Design review of the part built by this model. Coordinates are the model's own, in mm. A direction names the side the tool comes from. Coordinates: 2 decimals unless noted, no trailing zeros. Loops run counter-clockwise (first coordinate to the right, second up) from the corner with the lowest first, then second, coordinate; pieces in that order, holes last. Notation, with made-up numbers: M 15.5,-4 L 29.5,-4 A28 ccw 29.5,19 Z; hole C 83.5,86.5 d6. An arc over 180 degrees is marked long. Put each result on its own line as item: value. Start each with the question number.
(1) Take a section at A-A, the plane x = 8. Give the boundary of the cut face in (y, z).
(2) Take a section at C-C, the plane y = 10. Count the separate pieces of the cut face and the enclosed holes in it, then the cut area to 3 significant figures.
(3) Take a section at B-B, the plane x = 18. Give the boundary of the cut face in (y, z), then the cut area to 3 significant figures.
(4) Clearance check with flat-ended pins moving along their axes: pin 1 (1.5 mm diameter, centred on y = 10, z = -42.5, fed in from +X); pin 2 (6.5 mm diameter, centred on x = 8, z = -25, fed in from -Y); pin 3 (9 mm diameter, centred on y = 14.5, z = -23, fed in from +X); pin 4 (1.5 mm diameter, centred on x = 23.5, y = 7.5, fed in from -Z). State where each tip first meets the part, or that it passes through.
(5) For faces 4 (the flat face through (16, 17, -25)), 5 (the flat face through (6, 12, -23)), 6 (the flat face through (20, 12, -25)), 7 (the cylindrical face through (56.88, 5.42, -12.58)), list the 3-axis set-ups (+Z, -Z, +X, -X, +Y, -Y) from which the entire face can be reached by the end or side of a thin tool; tool diameter is ignored.
(6) The part is to be moulded in two halves that separate along Z. For faces 1 (the flat face through (27, 0, -25)), 2 (the cylindrical face through (18, 18.4, -41.9)), 3 (the flat face through (11, 10, 0)), say which applies: +Z half, -Z half, draft (parallel to the pull), parting line (faces both ways), or undercut.
(7) For probe 1 along X at (y, z) = (13.7, -25); probe 2 along Z at (x, y) = (13.5, 3.75); probe 3 along Y at (x, z) = (15.5, -21.5), list the stretches that pass through material, from the lowest coordinate up. Write a range as [from, to].
```python
from build123d import *

# Parameters (mm, degrees)
EXTRUDE_1_DEPTH             = 20
SKETCH_2_R                  = 7
CUT_EXTRUDE_1_DEPTH         = 20
SKETCH_3_R                  = 13
CUT_EXTRUDE_2_DEPTH         = 87.740993769
SKETCH_4_R                  = 16
CUT_EXTRUDE_3_DEPTH         = 19
CUT_EXTRUDE_9_DEPTH         = 87.740993769
EXTRUDE_START               = -20
EXTRUDE_4_DEPTH             = 20
FILLET_2_R                  = 3
SKETCH_7_R                  = 20.5
CUT_EXTRUDE_10_DEPTH        = 9
SKETCH_8_W                  = 29.8
SKETCH_8_H                  = 4
CUT_EXTRUDE_11_DEPTH        = 20
CUT_EXTRUDE_12_DEPTH        = 10
HOLE_WIZARD_M41_D           = 4.3
HOLE_WIZARD_M41_DEPTH       = 8
HOLE_WIZARD_M41_CBORE_D     = 8
HOLE_WIZARD_M41_CBORE_DEPTH = 4.5
M4X0_71_D                   = 3.3
HOLE_WIZARD_M31_D           = 3.2


# Read off the part's stored shape, not the designer's step: Бобышка-Вытянуть4
with BuildPart() as part:
    # Эскиз1 → Бобышка-Вытянуть1 (new body)
    with BuildSketch(Plane(origin=(0, 0, 0), x_dir=(1, 0, 0), z_dir=(0, 1, 0))):
        with BuildLine():
            Line((0, 0), (0, 50))
            Line((0, 50), (20, 50))
            Line((20, 50), (47.60878471, 47.400960405))
            ThreePointArc((47.60878471, 47.400960405), (68, 25), (47.60878471, 2.599039595))
            Line((47.60878471, 2.599039595), (20, 0))
            Line((20, 0), (0, 0))
        make_face()
    extrude(amount=EXTRUDE_1_DEPTH)

    # Эскиз2 → Вырез-Вытянуть1 (cut)
    with BuildSketch(Plane.ZY):
        with Locations((-39.9, 10)):
            Circle(SKETCH_2_R)
        with Locations(Location((-10.1, 10, 0), (0, 0, 180))):
            Circle(SKETCH_2_R)
    extrude(amount=-CUT_EXTRUDE_1_DEPTH, mode=Mode.SUBTRACT)

    # Эскиз3 → Вырез-Вытянуть2 (cut, through all)
    with BuildSketch(Plane(origin=(0, 20, 0), x_dir=(1, 0, 0), z_dir=(0, 1, 0))):
        with Locations(Location((45.5, 25, 0), (0, 0, 270))):
            Circle(SKETCH_3_R)
    extrude(amount=-CUT_EXTRUDE_2_DEPTH, mode=Mode.SUBTRACT)

    # Эскиз4 → Вырез-Вытянуть3 (cut)
    with BuildSketch(Plane(origin=(0, 20, 0), x_dir=(1, 0, 0), z_dir=(0, 1, 0))):
        with Locations(Location((45.5, 25, 0), (0, 0, 270))):
            Circle(SKETCH_4_R)
    extrude(amount=-CUT_EXTRUDE_3_DEPTH, mode=Mode.SUBTRACT)

    # Эскиз5 → Вырез-Вытянуть9 (cut, through all)
    with BuildSketch(Plane(origin=(0, 20, 0), x_dir=(1, 0, 0), z_dir=(0, 1, 0))):
        with BuildLine():
            add(Edge.make_bspline(
                [(47.32108314, 47.428044097), (47.41641101, 47.41948544), (47.512308925, 47.410461109), (47.60878471, 47.400960405)],
                knots=[0.992066387, 0.992066387, 0.992066387, 0.992066387, 1, 1, 1, 1], degree=3))
            Line((47.32108314, 47.428044095), (47.60878471, 47.400960405))
        make_face()
        with BuildLine():
            Line((47.32108314, 47.428044097), (23, 49.717585585))
            add(Edge.make_bspline(
                [(23, 49.717585585), (32.393861284, 42.286998451), (35.400716473, 48.498269788), (47.32108314, 47.428044097)],
                knots=[0, 0, 0, 0, 0.992066387, 0.992066387, 0.992066387, 0.992066387], degree=3))
        make_face()
        with BuildLine():
            add(Edge.make_bspline(
                [(23, 0.282414415), (32.393861284, 7.713001549), (35.400716473, 1.501730212), (47.32108314, 2.571955903)],
                knots=[0, 0, 0, 0, 0.992066387, 0.992066387, 0.992066387, 0.992066387], degree=3))
            Line((23, 0.282414415), (47.32108314, 2.571955903))
        make_face()
        with BuildLine():
            Line((47.60878471, 2.599039595), (47.32108314, 2.571955905))
            add(Edge.make_bspline(
                [(47.32108314, 2.571955903), (47.41641101, 2.58051456), (47.512308925, 2.589538891), (47.60878471, 2.599039595)],
                knots=[0.992066387, 0.992066387, 0.992066387, 0.992066387, 1, 1, 1, 1], degree=3))
        make_face()
    extrude(amount=-CUT_EXTRUDE_9_DEPTH, mode=Mode.SUBTRACT)

    # Бобышка-Вытянуть4 outline → Бобышка-Вытянуть4 (add)
    with BuildSketch(Plane(origin=(0, 20, 0), x_dir=(1, 0, 0), z_dir=(0, 1, 0)).offset(EXTRUDE_START)):
        with BuildLine():
            add(Edge.make_bspline(
                [(22.6429674, 50), (22.761978267, 49.905861862), (22.880989133, 49.811723723), (23, 49.717585585)],
                knots=[-0.012568493, -0.012568493, -0.012568493, -0.012568493, 0, 0, 0, 0], degree=3))
            Line((22.6429674, 50), (20, 50))
            Line((20, 50), (23, 49.717585585))
        make_face()
        with BuildLine():
            Line((20, 0), (22.6479861, 0))
            add(Edge.make_bspline(
                [(22.6479861, 0), (22.766323231, 0.09625734), (22.883651508, 0.190382227), (23, 0.282414415)],
                knots=[-0.012287325, -0.012287325, -0.012287325, -0.012287325, 0, 0, 0, 0], degree=3))
            Line((23, 0.282414415), (20, 0))
        make_face()
    extrude(amount=EXTRUDE_4_DEPTH)

    # Скругление2
    fillet_2_edges = [part.edges().sort_by_distance(p)[0] for p in [
        (11.32399305, 0, 0),
        (11.32399305, 20, 0),
        (11.3214837, 0, -50),
        (11.3214837, 20, -50),
    ]]
    fillet(fillet_2_edges, radius=FILLET_2_R)

    # Эскиз7 → Вырез-Вытянуть10 (cut)
    with BuildSketch(Plane(origin=(0, 20, 0), x_dir=(1, 0, 0), z_dir=(0, 1, 0))):
        with Locations(Location((45.5, 25, 0), (0, 0, 270))):
            Circle(SKETCH_7_R)
    extrude(amount=-CUT_EXTRUDE_10_DEPTH, mode=Mode.SUBTRACT)

    # Эскиз8 → Вырез-Вытянуть11 (cut)
    with BuildSketch(Plane.ZY):
        with Locations((-25, 10)):
            Rectangle(SKETCH_8_W, SKETCH_8_H)
    extrude(amount=-CUT_EXTRUDE_11_DEPTH, mode=Mode.SUBTRACT)

    # Эскиз9 → Вырез-Вытянуть12 (cut)
    with BuildSketch(Plane(origin=(0, 20, 0), x_dir=(1, 0, 0), z_dir=(0, 1, 0))):
        with BuildLine():
            Line((20, 39.9), (20, 10.1))
            ThreePointArc((20, 10.1), (18, 8.1), (16, 10.1))
            Line((16, 10.1), (16, 39.9))
            ThreePointArc((16, 39.9), (18, 41.9), (20, 39.9))
        make_face()
    extrude(amount=-CUT_EXTRUDE_12_DEPTH, mode=Mode.SUBTRACT)

    # Цековка для винта с внутренним шестигранником M41
    with Locations(Plane(origin=(0, 20, 0), x_dir=(1, 0, 0), z_dir=(0, 1, 0))):
        with Locations((8, 25)):
            CounterBoreHole(HOLE_WIZARD_M41_D / 2, HOLE_WIZARD_M41_CBORE_D / 2, HOLE_WIZARD_M41_CBORE_DEPTH, depth=HOLE_WIZARD_M41_DEPTH)

    # Отверстие обработанное метчиком M4x0.71 (through all)
    with Locations(Plane(origin=(0, 8, 0), x_dir=(1, 0, 0), z_dir=(0, 1, 0))):
        with Locations((8, 25)):
            Hole(M4X0_71_D / 2)

    # Отверстие с зазором M31 (through all)
    with Locations(Plane(origin=(0, 11, 0), x_dir=(1, 0, 0), z_dir=(0, 1, 0))):
        with Locations((32.595301243, 37.904698757), (58.404698757, 37.904698757), (58.404698757, 12.095301243), (32.595301243, 12.095301243)):
            Hole(HOLE_WIZARD_M31_D / 2)


solid = part.part
```
Computed values:
1. outline: M 0,-47 A3 ccw 3,-50 L 17,-50 A3 ccw 20,-47 L 20,-29 L 15.5,-29 L 15.5,-27.15 L 12,-27.15 L 12,-33.19 A7 cw long 8,-33.19 L 8,-26.65 L 0,-26.65 Z; M 0,-23.35 L 8,-23.35 L 8,-16.81 A7 cw long 12,-16.81 L 12,-22.85 L 15.5,-22.85 L 15.5,-21 L 20,-21 L 20,-3 A3 ccw 17,0 L 3,0 A3 ccw 0,-3 Z
2. separate pieces: 1
2. enclosed holes: 5
2. area: 1,220 mm^2
3. outline: M 0,-47 A3 ccw 3,-50 L 17,-50 A3 ccw 20,-47 L 20,-41.9 L 16.71,-41.9 A7 cw long 8,-33.19 L 8,-16.81 A7 cw long 16.71,-8.1 L 20,-8.1 L 20,-3 A3 ccw 17,0 L 3,0 A3 ccw 0,-3 Z
3. area: 419 mm^2
4. pin 1: stops at x = 60.52
4. pin 2: stops at y = 0
4. pin 3: stops at x = 68
4. pin 4: stops at z = -49.92
5. face 4: +Y
5. face 5: -X
5. face 6: none
5. face 7: +Y, -Y
6. face 1: draft
6. face 2: undercut
6. face 3: +Z half
7. probe 1: x = [0, 5.85], [10.15, 16], [20, 25], [66, 68]
7. probe 2: z = [-50, -43.05], [-36.75, -13.25], [-6.95, 0]
7. probe 3: y = [0, 8], [12, 20]
